CAD build for the part. Positions are in the model's coordinates, mm. Face numbers are marked on the shaded views. Round coordinates to 2 decimals unless told otherwise and drop trailing zeros. Order: outer loops, then holes, each group sorted by start corner. A loop starts at its lowest first (then second) coordinate and runs counter-clockwise, first axis right, second up. Notation, with made-up numbers: M -40,32 L -26,32 A17 cw -26,43 Z; hole C -30,-31 d9. An arc over 180 degrees is marked long. Answer as a JSON object with one key per item and string values.
```python
from build123d import *

# Parameters (mm, degrees)
SKETCH2_W             = 38.1
SKETCH2_H             = 16.7005
BOSS_EXTRUDE1_DEPTH   = 3.96875
F_8_CLEARANCE_HOLE1_D = 4.3053
CHAMFER1_SIZE         = 1.6002


with BuildPart() as part:
    # Sketch2 → Boss-Extrude1 (new body)
    with BuildSketch(Plane.XY):
        Rectangle(SKETCH2_W, SKETCH2_H)
    extrude(amount=BOSS_EXTRUDE1_DEPTH)

    # #8 Clearance Hole1 (through all)
    with Locations(Plane.XY.offset(3.96875)):
        with Locations((-11.1125, 0), (11.1125, 0)):
            Hole(F_8_CLEARANCE_HOLE1_D / 2)

    # Chamfer1
    chamfer1_edges = [part.edges().sort_by_distance(p)[0] for p in [
        (-19.05, 0, 3.96875),
        (0, -8.35025, 3.96875),
        (19.05, 0, 3.96875),
        (0, 8.35025, 3.96875),
    ]]
    chamfer(chamfer1_edges, length=CHAMFER1_SIZE)


solid = part.part
```
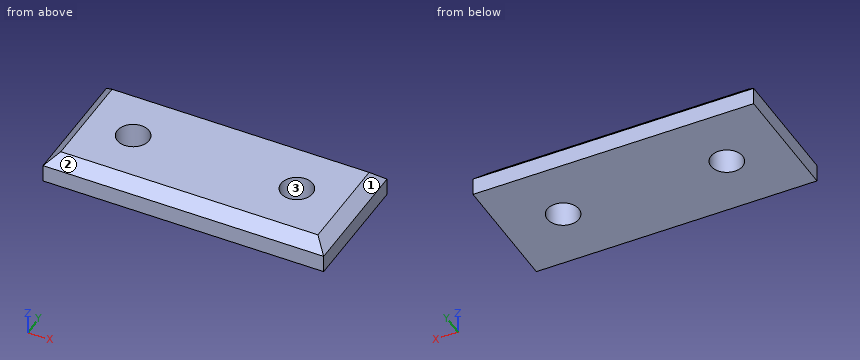
Item 1: Saw through at B-B on z = 1.6. List the corners of the cut face in (x, y), and give its area (3 significant figures).
Worked answers:
{"outline": "M -19.05,-8.35 L 19.05,-8.35 L 19.05,8.35 L -19.05,8.35 Z; hole C -11.11,0 d4.31; hole C 11.11,0 d4.31", "area": "607 mm2"}
Item 2: Saw through at A-A on y = 0. List the corners of the cut face in (x, z).
Worked answers:
{"outline": "M -19.05,0 L -13.27,0 L -13.27,3.97 L -17.45,3.97 L -19.05,2.37 Z; M -8.96,0 L 8.96,0 L 8.96,3.97 L -8.96,3.97 Z; M 13.27,0 L 19.05,0 L 19.05,2.37 L 17.45,3.97 L 13.27,3.97 Z"}
Item 3: Wall check: line 1 along X through (y, z) = (1.5, 3.85); line 2 along X through (y, z) = (0.25, 0.5); line 3 along Y through (x, z) = (12, 3.25). Give the ranges that are in metal, low to high. Write a range as [from, to].
Worked answers:
{"line 1": "x = [-17.57, -12.66], [-9.57, 9.57], [12.66, 17.57]", "line 2": "x = [-19.05, -13.25], [-8.97, 8.97], [13.25, 19.05]", "line 3": "y = [-7.47, -1.96], [1.96, 7.47]"}
Item 4: Saw through at D-D on y = -3.25. List the corners of the cut face in (x, z), and give its area (3 significant figures).
Worked answers:
{"outline": "M -19.05,0 L 19.05,0 L 19.05,2.37 L 17.45,3.97 L -17.45,3.97 L -19.05,2.37 Z", "area": "149 mm2"}
Item 5: Drop flat-ended pins along their axis: pin 1 Ø1 at (x, z) = (7, 3) entering from +Y; pin 2 Ø7 at (x, y) = (-11.11, 0) entering from +Z; pin 3 Ø1.5 at (y, z) = (-6.5, 3.5) entering from +X. Give the stop position or say it passes through.
Worked answers:
{"pin 1": "stops at y = 8.22", "pin 2": "stops at z = 3.97", "pin 3": "stops at x = 18.67"}
Item 6: Saw through at C-C on x = -7. List the corners of the cut face in (y, z).
Worked answers:
{"outline": "M -8.35,0 L 8.35,0 L 8.35,2.37 L 6.75,3.97 L -6.75,3.97 L -8.35,2.37 Z"}
Item 7: Two-plate mould, pull along X, no slides. Class the marked faces 1, 2 and 3: released by +X, released by -X, zero draft, split by the parting line, or undercut.
Worked answers:
{"face 1": "released by +X", "face 2": "zero draft", "face 3": "undercut"}
